```python
from build123d import *

# Parameters (mm, degrees)
CROQUIS2_W              = 1300
CROQUIS2_H              = 1000
SALIENTE_EXTRUIR1_DEPTH = 10
CROQUIS3_R              = 5
CORTAR_EXTRUIR1_DEPTH   = 11
CORTAR_EXTRUIR2_DEPTH   = 10
CORTAR_EXTRUIR3_DEPTH   = 10
CUT_EXTRUDE1_DEPTH      = 11


with BuildPart() as part:
    # Croquis2 → Saliente-Extruir1 (new body)
    with BuildSketch(Plane(origin=(0, 0, 0), x_dir=(1, 0, 0), z_dir=(0, 1, 0))):
        Rectangle(CROQUIS2_W, CROQUIS2_H)
    extrude(amount=SALIENTE_EXTRUIR1_DEPTH)

    # Croquis3 → Cortar-Extruir1 (cut, through all)
    with BuildSketch(Plane(origin=(0, 10, 0), x_dir=(1, 0, 0), z_dir=(0, 1, 0))):
        with Locations((-72.831998462, -137.867965644)):
            Circle(CROQUIS3_R)
        with Locations((33.234018716, -243.933982822)):
            Circle(CROQUIS3_R)
        with Locations((-72.831998462, -350)):
            Circle(CROQUIS3_R)
        with Locations((-178.89801564, -243.933982822)):
            Circle(CROQUIS3_R)
        with Locations((-461.740728115, 251.040764009)):
            Circle(CROQUIS3_R)
        with Locations((-355.674710937, 144.974746831)):
            Circle(CROQUIS3_R)
        with Locations((-461.740728115, 38.908729653)):
            Circle(CROQUIS3_R)
        with Locations((-567.806745293, 144.974746831)):
            Circle(CROQUIS3_R)
    extrude(amount=-CORTAR_EXTRUIR1_DEPTH, mode=Mode.SUBTRACT)

    # Croquis5 → Cortar-Extruir2 (cut)
    with BuildSketch(Plane(origin=(0, 0, 0), x_dir=(1, 0, 0), z_dir=(0, 1, 0))):
        Polygon((0, 0), (-500, 500), (650, 500), (650, -500), (500, -500), align=None)
        Polygon((-41.541714007, -500), (-650, 108.458285993), (-650, -500), align=None)
    extrude(amount=CORTAR_EXTRUIR2_DEPTH, mode=Mode.SUBTRACT)

    # Croquis6 → Cortar-Extruir3 (cut)
    with BuildSketch(Plane(origin=(0, 0, 0), x_dir=(1, 0, 0), z_dir=(0, 1, 0))):
        Polygon((-650, 108.458285993), (-379.229142997, 379.229142997), (-500, 500), (-650, 500), align=None)
        Polygon((-41.541714007, -500), (229.229142997, -229.229142997), (500, -500), align=None)
    extrude(amount=CORTAR_EXTRUIR3_DEPTH, mode=Mode.SUBTRACT)

    # Sketch1 → Cut-Extrude1 (cut, through all)
    with BuildSketch(Plane(origin=(0, 10, 0), x_dir=(1, 0, 0), z_dir=(0, 1, 0))):
        Polygon((-379.229142997, 379.229142997), (-469.383041958, 289.075244036), (139.075244036, -319.383041958), (229.229142997, -229.229142997), align=None)
    extrude(amount=-CUT_EXTRUDE1_DEPTH, mode=Mode.SUBTRACT)


solid = part.part
```
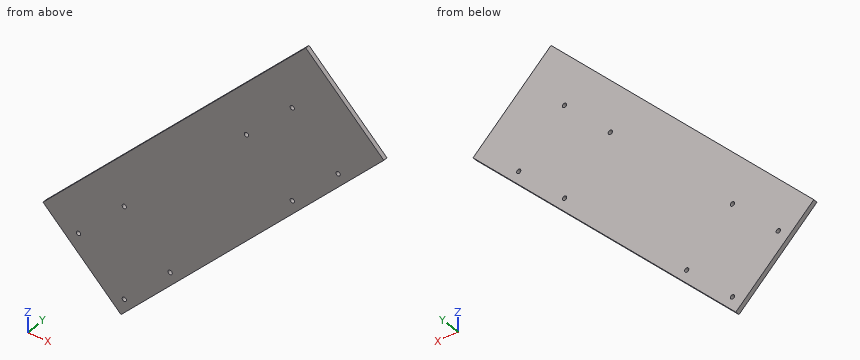
Can you work these out from the model? Positions are in its coordinate system, mm. Give positions to 0.01 mm unless a question says otherwise; leave off trailing zeros. Order: outer loops, then holes, each group sorted by start corner. A loop starts at its lowest first (then second) coordinate and runs counter-clockwise, first axis right, second up. Notation, with made-up numbers: M 51,-11.5 L 88,-11.5 A28 cw 88,10.5 Z; hole C 55,-28 d5. An arc over 180 degrees is marked long. Write item = value, one per line. Start each with the question number.
Q1. I need wall thicknesses on probe 1 along Z at (x, y) = (-69.5, 7); probe 2 along X at (y, z) = (1.5, 124); probe 3 along X at (y, z) = (5.75, 233.5). Which ranges of each line are inside material? Lowest first, please. Write a range as [from, to].
Q2. Will these pins go through, and if not, where does the flat tip stop? pin 1 Ø1 at (x, y) = (-214, 6.5) entering from +Z; pin 2 Ø16 at (x, z) = (33.23, 243.93) entering from -Y; pin 3 Ø6 at (x, z) = (-72.83, 350) entering from -Y; pin 4 Ø1.5 at (y, z) = (2, 242.5) entering from +X.
Q3. Suppose I cut it at B-B (x = -267.5). Write out the boundary of the cut face in (y, z), plus the area to 3 significant figures.
Q4. Suppose I cut it at C-C (z = -2). Write out the boundary of the cut face in (x, y).
Q5. Suppose I cut it at A-A (y = 4.75). Count the separate pieces of the cut face and the enclosed holes in it, plus the area to 3 significant figures.
Check result:
q1.probe_1 = [110.81, 134.14], [141.6, 346.27], [353.73, 472.04]
q1.probe_2 = [-417.54, -56.31]
q1.probe_3 = [-308.04, 53.19]
q2.pin_1 = 328.04
q2.pin_2 = 0
q2.pin_3 = through
q2.pin_4 = 62.94
q3.outline = M 0,-87.19 L 10,-87.19 L 10,274.04 L 0,274.04 Z
q3.area = 3,610 mm2
q4.outline = M -543.54,0 L -182.31,0 L -182.31,10 L -543.54,10 Z
q5.separate_pieces = 1
q5.enclosed_holes = 8
q5.area = 219,000 mm2
